```python
from build123d import *

# Parameters (mm, degrees)
SKETCH1_W           = 100
SKETCH1_H           = 18
SKETCH1_W_2         = 18
SKETCH1_H_2         = 100
BOSS_EXTRUDE1_DEPTH = 18


with BuildPart() as part:
    # Sketch1 → Boss-Extrude1 (new body)
    with BuildSketch(Plane.XY):
        with BuildLine():
            Line((-817.41132124, 1115.015948799), (-417.41132124, 1115.015948799))
            ThreePointArc((-417.41132124, 1115.015948799), (-346.700643121, 1085.726626917), (-317.41132124, 1015.015948799))
            Line((-317.41132124, 1015.015948799), (-317.41132124, 415.015948799))
            Line((-317.41132124, 415.015948799), (-817.41132124, 415.015948799))
            Line((-817.41132124, 415.015948799), (-817.41132124, 1115.015948799))
        make_face()
        with Locations((-667.41132124, 430.015948799)):
            Rectangle(SKETCH1_W, SKETCH1_H, mode=Mode.SUBTRACT)
        with Locations((-467.41132124, 580.015948799)):
            Rectangle(SKETCH1_W, SKETCH1_H, mode=Mode.SUBTRACT)
        with Locations((-467.41132124, 430.015948799)):
            Rectangle(SKETCH1_W, SKETCH1_H, mode=Mode.SUBTRACT)
        with Locations((-667.41132124, 580.015948799)):
            Rectangle(SKETCH1_W, SKETCH1_H, mode=Mode.SUBTRACT)
        with Locations((-467.41132124, 730.015948799)):
            Rectangle(SKETCH1_W, SKETCH1_H, mode=Mode.SUBTRACT)
        with Locations((-667.41132124, 730.015948799)):
            Rectangle(SKETCH1_W, SKETCH1_H, mode=Mode.SUBTRACT)
        with Locations((-467.41132124, 880.015948799)):
            Rectangle(SKETCH1_W, SKETCH1_H, mode=Mode.SUBTRACT)
        with Locations((-667.41132124, 880.015948799)):
            Rectangle(SKETCH1_W, SKETCH1_H, mode=Mode.SUBTRACT)
        with Locations((-802.41132124, 495.015948799)):
            Rectangle(SKETCH1_W_2, SKETCH1_H_2, mode=Mode.SUBTRACT)
        with Locations((-802.41132124, 1035.015948799)):
            Rectangle(SKETCH1_W_2, SKETCH1_H_2, mode=Mode.SUBTRACT)
    extrude(amount=BOSS_EXTRUDE1_DEPTH)


solid = part.part
```
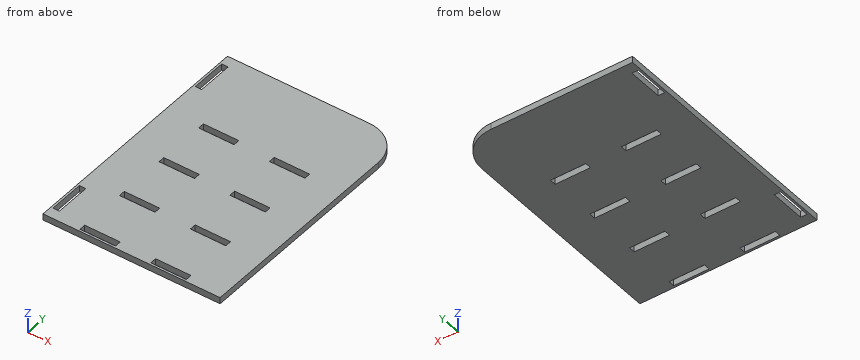
Part model, mm, in its own coordinate system. Round coordinates to 2 decimals unless told otherwise and drop trailing zeros. Order: outer loops, then holes, each group sorted by start corner. A loop starts at its lowest first (then second) coordinate and runs counter-clockwise, first axis right, second up. Notation, with made-up numbers: M 69.25,89.25 L 87.25,89.25 A15 cw 87.25,95.25 Z; hole C -28,44.25 d5. An arc over 180 degrees is marked long. Answer in a Markdown table with one row per item. Add a question column.
Q1. Wall check: L1, parallel to X at y = 587.5, z = 2.25; L2, parallel to Y at x = -707, z = 9; L3, parallel to X at y = 490, z = 9.25. Give the ranges that are in metal, low to high. Write a range as from..to.
Q2. Cut at D-D on z = 9.25. Give the number of separate pieces and of enclosed holes in the cut face, and give its area (3 significant figures).
Q3. Cut at A-A on x = -666.5. Give the cut face in (y, z).
Q4. Cut at B-B on y = 731. Give the cut face in (x, z), and give its area (3 significant figures).
Q5. Cut at C-C on y = 533. Give the cut face in (x, z), and give its area (3 significant figures).
Established:
| question | item | result |
|---|---|---|
| 1 | L1 | x = -817.41..-717.41, -617.41..-517.41, -417.41..-317.41 |
| 1 | L2 | y = 415.02..421.02, 439.02..571.02, 589.02..721.02, 739.02..871.02, 889.02..1115.02 |
| 1 | L3 | x = -817.41..-811.41, -793.41..-317.41 |
| 2 | separate pieces | 1 |
| 2 | enclosed holes | 10 |
| 2 | area | 330,000 mm2 |
| 3 | outline | M 415.02,0 L 421.02,0 L 421.02,18 L 415.02,18 Z; M 439.02,0 L 571.02,0 L 571.02,18 L 439.02,18 Z; M 589.02,0 L 721.02,0 L 721.02,18 L 589.02,18 Z; M 739.02,0 L 871.02,0 L 871.02,18 L 739.02,18 Z; M 889.02,0 L 1115.02,0 L 1115.02,18 L 889.02,18 Z |
| 4 | outline | M -817.41,0 L -717.41,0 L -717.41,18 L -817.41,18 Z; M -617.41,0 L -517.41,0 L -517.41,18 L -617.41,18 Z; M -417.41,0 L -317.41,0 L -317.41,18 L -417.41,18 Z |
| 4 | area | 5,400 mm2 |
| 5 | outline | M -817.41,0 L -811.41,0 L -811.41,18 L -817.41,18 Z; M -793.41,0 L -317.41,0 L -317.41,18 L -793.41,18 Z |
| 5 | area | 8,680 mm2 |
